```python
from build123d import *

# Parameters (mm, degrees)
F0_R         = 12.5
F1_DEPTH     = 12.5
F2_R         = 2.25
F3_DEPTH     = 25
F4_R         = 12.5
F5_DEPTH     = 7.5
F6_T1_DEPTH  = 24.050587715
F6_T3_DEPTH  = 24.050587715
F6_T5_DEPTH  = 24.050587715
F6_T7_DEPTH  = 24.050587715
F6_T9_DEPTH  = 24.050587715
F6_T11_DEPTH = 24.050587715
F6_T13_DEPTH = 24.050587715
F8_DEPTH     = 2


# Not quite as in the source:
# - a fillet or chamfer that OpenCascade refuses, or shapes differently, is made with other operations: its cross-section is extruded or revolved along the edge and cut away or added


with BuildPart() as f1:
    # F0 (on Top) → F1 (new body, symmetric)
    with BuildSketch(Plane.XY):
        Polygon((22.5, -5.1354781738), (22.5, 5.1354781738), (18.0435990556, 14.3892900865), (10.013442028, 20.7931266245), (0, 23.0786294236), (-10.013442028, 20.7931266245), (-18.0435990556, 14.3892900865), (-22.5, 5.1354781738), (-22.5, -5.1354781738), (-18.0435990556, -14.3892900865), (-10.013442028, -20.7931266245), (0, -23.0786294236), (10.013442028, -20.7931266245), (18.0435990556, -14.3892900865), align=None)
        Circle(F0_R, mode=Mode.SUBTRACT)
    extrude(amount=F1_DEPTH, both=True)

    # F2 (on face) → F3 (cut)
    with BuildSketch(Plane.XY.offset(12.5)):
        with Locations((9, 15.5884572681)):
            Circle(F2_R)
        with Locations((-18, 0)):
            Circle(F2_R)
        with Locations((9, -15.5884572681)):
            Circle(F2_R)
    extrude(amount=-F3_DEPTH, mode=Mode.SUBTRACT)

    # F4 (on face) → F5 (join)
    with BuildSketch(Plane.XY.offset(12.5)):
        Polygon((14.35, -3.2752938575), (14.35, 3.2752938575), (11.5078065088, 9.1771694552), (6.3863508045, 13.2613940917), (0, 14.719036988), (-6.3863508045, 13.2613940917), (-11.5078065088, 9.1771694552), (-14.35, 3.2752938575), (-14.35, -3.2752938575), (-11.5078065088, -9.1771694552), (-6.3863508045, -13.2613940917), (0, -14.719036988), (6.3863508045, -13.2613940917), (11.5078065088, -9.1771694552), align=None)
        Circle(F4_R, mode=Mode.SUBTRACT)
    extrude(amount=F5_DEPTH)

    # F6: fillet of radius 3.5 on 7 edges, made by hand

    # F6_s2 → F6_t1 (cut)
    with BuildSketch(Plane.XZ.offset(-12.0252938575)):
        with BuildLine():
            ThreePointArc((-10.85, 20), (-13.3248737342, 18.9748737342), (-14.35, 16.5))
            Line((-14.35, 16.5), (-14.35, 20))
            Line((-14.35, 20), (-10.85, 20))
        make_face()
    extrude(amount=F6_T1_DEPTH, mode=Mode.SUBTRACT)

    # F6_s4 → F6_t3 (cut)
    with BuildSketch(Plane(origin=(-9.4017533237, 7.4976480845, 0), x_dir=(0, 0, 1), z_dir=(0.7818314825, -0.6234898019, 0))):
        with BuildLine():
            ThreePointArc((20, 10.85), (18.9748737342, 13.3248737342), (16.5, 14.35))
            Line((16.5, 14.35), (20, 14.35))
            Line((20, 14.35), (20, 10.85))
        make_face()
    extrude(amount=F6_T3_DEPTH, mode=Mode.SUBTRACT)

    # F6_s6 → F6_t5 (cut)
    with BuildSketch(Plane(origin=(-11.7237946339, -2.6758796203, 0), x_dir=(0, 0, 1), z_dir=(0.9749279122, 0.222520934, 0))):
        with BuildLine():
            ThreePointArc((20, 10.85), (18.9748737342, 13.3248737342), (16.5, 14.35))
            Line((16.5, 14.35), (20, 14.35))
            Line((20, 14.35), (20, 10.85))
        make_face()
    extrude(amount=F6_T5_DEPTH, mode=Mode.SUBTRACT)

    # F6_s8 → F6_t7 (cut)
    with BuildSketch(Plane(origin=(-5.2175794629, -10.834415393, 0), x_dir=(0, 0, 1), z_dir=(0.4338837391, 0.9009688679, 0))):
        with BuildLine():
            ThreePointArc((20, 10.85), (18.9748737342, 13.3248737342), (16.5, 14.35))
            Line((16.5, 14.35), (20, 14.35))
            Line((20, 14.35), (20, 10.85))
        make_face()
    extrude(amount=F6_T7_DEPTH, mode=Mode.SUBTRACT)

    # F6_s10 → F6_t9 (cut)
    with BuildSketch(Plane(origin=(5.2175794629, -10.834415393, 0), x_dir=(0, 0, 1), z_dir=(-0.4338837391, 0.9009688679, 0))):
        with BuildLine():
            ThreePointArc((20, 10.85), (18.9748737342, 13.3248737342), (16.5, 14.35))
            Line((16.5, 14.35), (20, 14.35))
            Line((20, 14.35), (20, 10.85))
        make_face()
    extrude(amount=F6_T9_DEPTH, mode=Mode.SUBTRACT)

    # F6_s12 → F6_t11 (cut)
    with BuildSketch(Plane(origin=(11.7237946339, -2.6758796203, 0), x_dir=(0, 0, 1), z_dir=(-0.9749279122, 0.222520934, 0))):
        with BuildLine():
            ThreePointArc((20, 10.85), (18.9748737342, 13.3248737342), (16.5, 14.35))
            Line((16.5, 14.35), (20, 14.35))
            Line((20, 14.35), (20, 10.85))
        make_face()
    extrude(amount=F6_T11_DEPTH, mode=Mode.SUBTRACT)

    # F6_s14 → F6_t13 (cut)
    with BuildSketch(Plane(origin=(9.4017533237, 7.4976480845, 0), x_dir=(0, 0, 1), z_dir=(-0.7818314825, -0.6234898019, 0))):
        with BuildLine():
            ThreePointArc((20, 10.85), (18.9748737342, 13.3248737342), (16.5, 14.35))
            Line((16.5, 14.35), (20, 14.35))
            Line((20, 14.35), (20, 10.85))
        make_face()
    extrude(amount=F6_T13_DEPTH, mode=Mode.SUBTRACT)

    # F7 (on face) → F8 (cut)
    with BuildSketch(Plane.YZ.offset(22.5)):
        with BuildLine():
            ThreePointArc((-6.08032713, 7), (-6.5709395266, 5.8842188275), (-6.8446164746, 4.6964608232))
            add(Edge.make_bspline(
                [(-6.8446164746, 4.6964608232), (-8.5118431653, 3.8987596156), (-7.5942066586, 1.756193723), (-6.676570152, -0.3863721695), (-5.4204160797, 1.3711319286), (-4.1642620074, 3.1286360267), (-5.6446164746, 4.4838947381)],
                knots=[3.4647722977, 3.4647722977, 3.4647722977, 5.2614695117, 5.2614695117, 7.0581667257, 7.0581667257, 8.8548639397, 8.8548639397, 8.8548639397], degree=2, weights=[1, 0.6229027007, 1, 0.6229027007, 1, 0.6229027007, 1]))
            ThreePointArc((-5.6446164746, 4.4838947381), (-5.761433535, 5.7594440336), (-6.08032713, 7))
        make_face()
        with BuildLine():
            ThreePointArc((-3, 8), (-3.6341058947, 6.5649040102), (-3.9, 5.0186533479))
            add(Edge.make_bspline(
                [(-3.9, 5.0186533479), (-5.3449244407, 3.7673120757), (-4.2724622204, 1.8501460197), (-3.2, -0.0670200364), (-2.1275377796, 1.8501460197), (-1.0550755593, 3.7673120757), (-2.5, 5.0186533479)],
                knots=[3.6651914292, 3.6651914292, 3.6651914292, 5.4105206812, 5.4105206812, 7.1558499332, 7.1558499332, 8.9011791852, 8.9011791852, 8.9011791852], degree=2, weights=[1, 0.6427876097, 1, 0.6427876097, 1, 0.6427876097, 1]))
            ThreePointArc((-2.5, 5.0186533479), (-2.5591609645, 6.5413321832), (-3, 8))
        make_face()
        with BuildLine():
            ThreePointArc((0.2275558291, 8.2), (-0.3814401497, 6.9183905981), (-0.6724441709, 5.5296086062))
            add(Edge.make_bspline(
                [(-0.6724441709, 5.5296086062), (-4.5551319088, 2.1883602337), (-0.1559076785, 1.4136843578), (4.2433165517, 0.6390084818), (0.9275558291, 5.247858612)],
                knots=[3.6426090527, 3.6426090527, 3.6426090527, 6.1715912058, 6.1715912058, 8.7005733589, 8.7005733589, 8.7005733589], degree=2, weights=[1, 0.301537928, 1, 0.301537928, 1]))
            ThreePointArc((0.9275558291, 5.247858612), (0.7672369702, 6.7689057422), (0.2275558291, 8.2))
        make_face()
        with BuildLine():
            ThreePointArc((4.6275558291, 7.5), (3.6127003085, 6.4223734822), (2.8925635541, 5.1290778105))
            add(Edge.make_bspline(
                [(2.8925635541, 5.1290778105), (-1.6007345704, 2.6680437483), (2.6559421174, 1.1765704347), (6.9126188052, -0.3149028789), (4.4025558291, 4.6)],
                knots=[3.6564949123, 3.6564949123, 3.6564949123, 6.1933168635, 6.1933168635, 8.7301388146, 8.7301388146, 8.7301388146], degree=2, weights=[1, 0.2977981768, 1, 0.2977981768, 1]))
            ThreePointArc((4.4025558291, 4.6), (4.6934507475, 6.036159015), (4.6275558291, 7.5))
        make_face()
        with BuildLine():
            ThreePointArc((7.8275558291, 2.635071483), (6.9777355341, 1.9893158846), (6.3875558291, 1.1))
            add(Edge.make_bspline(
                [(6.3875558291, 1.1), (0.8266327144, -0.0014683083), (5.3606005397, -2.5921173467), (9.8945683651, -5.182766385), (7.6126455386, 0.4)],
                knots=[3.5803471544, 3.5803471544, 3.5803471544, 6.1960920441, 6.1960920441, 8.8118369337, 8.8118369337, 8.8118369337], degree=2, weights=[1, 0.2599050592, 1, 0.2599050592, 1]))
            ThreePointArc((7.6126455386, 0.4), (7.89881342, 1.5003518589), (7.8275558291, 2.635071483))
        make_face()
        with BuildLine():
            ThreePointArc((2.4, -9), (5.354892815, -9.90978563), (6.4, -7))
            ThreePointArc((6.4, -7), (0.8632403752, -1.8350585765), (-6.5, -3.6))
            ThreePointArc((-6.5, -3.6), (-6.8228285121, -5.9063339911), (-4.6, -6.6009044571))
            ThreePointArc((-4.6, -6.6009044571), (-0.6410576804, -6.4613658189), (2.4, -9))
        make_face()
    extrude(amount=-F8_DEPTH, mode=Mode.SUBTRACT)


solid = f1.part
```
Part model, mm, in its own coordinate system. A direction names the side the tool comes from. Coordinates: 2 decimals unless noted, no trailing zeros. Order: outer loops, then holes, each group sorted by start corner. A loop starts at its lowest first (then second) coordinate and runs counter-clockwise, first axis right, second up. Notation, with made-up numbers: (2.5, 32) -> (14.5, 32) arc R29 cw to (14.5, 64) -> close; hole circle Ø8 at (-22.75, -11). An arc over 180 degrees is marked (long way). Put each result on its own line as item: value. Start each with the question number.
(1) Band-saw the part on A-A (z = 15). Give the cut face in (x, y).
(2) Which spindle directions (+Z, -Z, +X, -X, +Y, -Y) get a long thin tool onto all of the face, cutting with end or side? Do faces 1 (the face through (-3.24, -13.98, 15.86)), 2 (the face through (-12.91, 6.27, 15.86)), 3 (the face through (3.24, 13.98, 14.47)). Say none if no direction does.
(3) Probe line 1 along Y through (x, z) = (9, -4); line 2 along Z through (x, y) = (-19.5, -2.5); line 3 along X through (y, z) = (0, 13). List the from-to ranges inside material, lowest first. Write a range as [from, to].
(4) Pin check, flat tips, straight feed: pin 1 Ø1.4 at (y, z) = (0, 4.5) entering from +X; pin 2 Ø6 at (x, y) = (9, -15.59) entering from -Z; pin 3 Ø15 at (x, y) = (0, 0) entering from -Z; pin 4 Ø5 at (x, y) = (-18, 0) entering from +Z. Stop position of each tip, or through.
(5) Mould opens along Z. For faces 4 (the face through (-20.3, -9.7, 0.2)), 5 (the face through (21.51, 0.77, 6.75)), 6 (the face through (21.514, -3.628, 6.586)), 7 (the face through (-8.45, -10.456, 18.851)) say: pulls with the +Z half, pulls with the -Z half, needs draft (parallel to the pull), parting line crosses it, or undercut.
Determined:
1. outline: (-14.35, -3.28) -> (-11.51, -9.18) -> (-6.39, -13.26) -> (0, -14.72) -> (6.39, -13.26) -> (11.51, -9.18) -> (14.35, -3.28) -> (14.35, 3.28) -> (11.51, 9.18) -> (6.39, 13.26) -> (0, 14.72) -> (-6.39, 13.26) -> (-11.51, 9.18) -> (-14.35, 3.28) -> close; hole circle Ø25 at (0, 0)
2. face 1: +Z, -X, -Y
2. face 2: +Z, -X, +Y
2. face 3: +Z, +X, +Y
3. line 1: y = [-21.02, -17.84], [-13.34, -8.67], [8.67, 13.34], [17.84, 21.02]
3. line 2: z = [-12.5, 12.5]
3. line 3: x = [-14.35, -12.5], [12.5, 14.35]
4. pin 1: stops at x = 20.5
4. pin 2: stops at z = -12.5
4. pin 3: passes through
4. pin 4: stops at z = 12.5
5. face 4: needs draft
5. face 5: undercut
5. face 6: undercut
5. face 7: pulls with the +Z half
